Here's how the part is built. I have some questions about the finished solid (model axes, mm). A direction names the side the tool comes from. Round coordinates to 2 decimals unless told otherwise and drop trailing zeros. Order: outer loops, then holes, each group sorted by start corner. A loop starts at its lowest first (then second) coordinate and runs counter-clockwise, first axis right, second up.
```python
from build123d import *

# Parameters (mm, degrees)
SKETCH1_W           = 42
SKETCH1_H           = 42
SKETCH1_R           = 1.6
SKETCH1_R_2         = 5
BOSS_EXTRUDE1_DEPTH = 2
FILLET1_R           = 5


with BuildPart() as part:
    # Sketch1 → Boss-Extrude1 (new body)
    with BuildSketch(Plane(origin=(0, 0, 0), x_dir=(1, 0, 0), z_dir=(0, 1, 0))):
        Rectangle(SKETCH1_W, SKETCH1_H)
        with Locations(Location((15.5, 15.5, 0), (0, 0, 270))):
            Circle(SKETCH1_R, mode=Mode.SUBTRACT)
        with Locations(Location((-15.5, 15.5, 0), (0, 0, 90))):
            Circle(SKETCH1_R, mode=Mode.SUBTRACT)
        with Locations(Location((15.5, -15.5, 0), (0, 0, 90))):
            Circle(SKETCH1_R, mode=Mode.SUBTRACT)
        with Locations(Location((-15.5, -15.5, 0), (0, 0, 270))):
            Circle(SKETCH1_R, mode=Mode.SUBTRACT)
        with Locations(Location((0, 13, 0), (0, 0, 270))):
            Circle(SKETCH1_R_2, mode=Mode.SUBTRACT)
        with Locations(Location((13, 0, 0), (0, 0, 270))):
            Circle(SKETCH1_R_2, mode=Mode.SUBTRACT)
        with Locations(Location((0, -13, 0), (0, 0, 270))):
            Circle(SKETCH1_R_2, mode=Mode.SUBTRACT)
        with Locations(Location((-13, 0, 0), (0, 0, 270))):
            Circle(SKETCH1_R_2, mode=Mode.SUBTRACT)
        with BuildLine():
            Line((-2.5, 2.6), (2.5, 2.6))
            ThreePointArc((2.5, 2.6), (5.1, 0), (2.5, -2.6))
            Line((2.5, -2.6), (-2.5, -2.6))
            ThreePointArc((-2.5, -2.6), (-5.1, 0), (-2.5, 2.6))
        make_face(mode=Mode.SUBTRACT)
    extrude(amount=BOSS_EXTRUDE1_DEPTH)

    # Fillet1
    fillet1_edges = [part.edges().sort_by_distance(p)[0] for p in [
        (21, 1, 21),
        (-21, 1, 21),
        (-21, 1, -21),
        (21, 1, -21),
    ]]
    fillet(fillet1_edges, radius=FILLET1_R)


solid = part.part
```
1. If we section it at A-A, the plane x = -13: Write out the boundary of the cut face in (y, z), and give its area (3 significant figures).
Evaluation:
outline: (0, -21) - (2, -21) - (2, -5) - (0, -5) - close; (0, 5) - (2, 5) - (2, 21) - (0, 21) - close
area: 64.0 mm2
2. I'm going to push a flat-ended pin straight in: P1, Ø3, axis at x = 15.5, z = 15.5, coming from the -Y side. Where does the tip first touch, or does it pass through?
Evaluation:
P1: passes through
3. On a 3-axis mill with a long thin cutter (end or side, diameter ignored), from which of +Z, -Z, +X, -X, +Y, -Y can I reach the whole of each face in a straight line? I mean faces 5 (the cylindrical face through (-20, 1, 19)), 6 (the flat face through (0, 1, 2.6)). Say none if no direction works.
Evaluation:
face 5: +Z, -X, +Y, -Y
face 6: +Y, -Y
4. If we section it at B-B, the plane y = 1.2: State how many separate pieces and enclosed holes the cut face has, and give its area (3 significant figures).
Evaluation:
separate pieces: 1
enclosed holes: 9
area: 1,350 mm2
5. If we section it at D-D, the plane x = 0: Write out the boundary of the cut face in (y, z), and give its area (3 significant figures).
Evaluation:
outline: (0, -21) - (2, -21) - (2, -18) - (0, -18) - close; (0, -8) - (2, -8) - (2, -2.6) - (0, -2.6) - close; (0, 2.6) - (2, 2.6) - (2, 8) - (0, 8) - close; (0, 18) - (2, 18) - (2, 21) - (0, 21) - close
area: 33.6 mm2
6. I need wall thicknesses on probe 1 along X at (y, z) = (0.55, 0); probe 2 along X at (y, z) = (1.75, -16.5); probe 3 along Z at (x, y) = (2, 0.35). Which ranges of each line are inside material? Lowest first, please.
Evaluation:
probe 1: x = -21 to -18, -8 to -5.1, 5.1 to 8, 18 to 21
probe 2: x = -20.97 to -16.75, -14.25 to -3.57, 3.57 to 14.25, 16.75 to 20.97
probe 3: z = -21 to -17.58, -8.42 to -2.6, 2.6 to 8.42, 17.58 to 21
7. If we mould it in two halves opening along Z, with no side actions, what happens to faces 1 (the cylindrical face through (14.42, 0.99, 16.68)), 2 (the cylindrical face through (19, 1, 20)), 3 (the flat face through (0, 2, -5)), 4 (the cylindrical face through (-5.1, 1, 0.1))? For each: released by +Z, released by -Z, zero draft, split by the parting line, or undercut.
Evaluation:
face 1: undercut
face 2: released by +Z
face 3: zero draft
face 4: undercut
8. If we section it at C-C, the plane z = 16.5: Write out the boundary of the cut face in (x, y).
Evaluation:
outline: (-20.97, 0) - (-16.75, 0) - (-16.75, 2) - (-20.97, 2) - close; (-14.25, 0) - (-3.57, 0) - (-3.57, 2) - (-14.25, 2) - close; (3.57, 0) - (14.25, 0) - (14.25, 2) - (3.57, 2) - close; (16.75, 0) - (20.97, 0) - (20.97, 2) - (16.75, 2) - close
